Can you work these out from the model? Positions are in its coordinate system, mm. Face numbers are marked on the shaded views. Coordinates: 2 decimals unless noted, no trailing zeros. Loops run counter-clockwise (first coordinate to the right, second up) from the corner with the lowest first, then second, coordinate; pieces in that order, holes last.
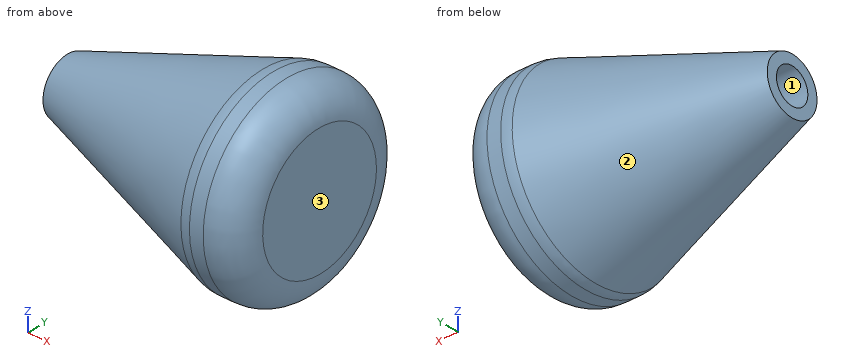
```python
from build123d import *

# Parameters (mm, degrees)
FILLET1_R = 5
FILLET2_R = 5


with BuildPart() as part:
    # Sketch1 → Revolve1 (revolve)
    with BuildSketch(Plane(origin=(0, 0, 0), x_dir=(0, 1, 0), z_dir=(0, 0, 1)), mode=Mode.PRIVATE) as revolve1_sk:
        Polygon((0, 0), (0, 6), (2.8, 6), (2.8, 40), (4.437898451, 40), (15.149054344, 8), (15.149054344, 0), align=None)
    revolve(revolve1_sk.sketch.rotate(Axis((0, 0, 0), (-1, 0, 0)), 90), axis=Axis((0, 0, 0), (-1, 0, 0)))

    # Fillet1
    fillet1_edges = [part.edges().sort_by_distance(p)[0] for p in [
        (-8, 0, 15.149054344),
    ]]
    fillet(fillet1_edges, radius=FILLET1_R)

    # Fillet2
    fillet2_edges = [part.edges().sort_by_distance(p)[0] for p in [
        (0, 0, 15.149054344),
    ]]
    fillet(fillet2_edges, radius=FILLET2_R)


solid = part.part
```
Item 1: Suppose I cut it at C-C, the plane x = -1.5. Please give me the cut outline in (y, z), plus the area to 3 significant figures.
Results are:
outline: circle Ø27.44 at (0, 0)
area: 591 mm2
Item 2: I'm going to push flat-ended pins straight in: P1, Ø1.5, axis at x = -20, y = 0, coming from the +Z side; P2, Ø8, axis at x = -25.5, z = -3.5, coming from the -Y side; P3, Ø1.7, axis at y = -1, z = 0.5, coming from the -X side. Where does each tip first touch, or does it pass through?
Results are:
P1: stops at z = 11.38
P2: stops at y = -10.35
P3: stops at x = -6
Item 3: Suppose I cut it at B-B, the plane x = -6.5. Please give me the cut outline in (y, z).
Results are:
outline: circle Ø30.3 at (0, 0); hole circle Ø5.6 at (0, 0)
Item 4: I need wall thicknesses on line 1 along Y through (x, z) = (-27, 0); line 2 along Y through (x, z) = (-28, 0); line 3 along X through (y, z) = (-9, 9). Which ranges of each line are inside material? Lowest first, please.
Results are:
line 1: y = -8.79 to -2.8, 2.8 to 8.79
line 2: y = -8.45 to -2.8, 2.8 to 8.45
line 3: x = -15.23 to -0.72
Item 5: We'd pull the mould along Y, two halves only. Please class the marked faces 1, 2 and 3: +Y half, -Y half, draft (parallel to the pull), parting line (faces both ways), or undercut.
Results are:
face 1: undercut
face 2: parting line
face 3: draft
Item 6: Suppose I cut it at A-A, the plane x = -11.5. Please give me the cut outline in (y, z).
Results are:
outline: circle Ø27.96 at (0, 0); hole circle Ø5.6 at (0, 0)
